Could you check a few things on this model? Use its own coordinates, in mm. A direction names the side the tool comes from. Give positions to 0.01 mm unless a question says otherwise; leave off trailing zeros. Order: outer loops, then holes, each group sorted by start corner. A loop starts at its lowest first (then second) coordinate and runs counter-clockwise, first axis right, second up. Notation, with made-up numbers: (-4.75, -21.5) -> (41.25, -21.5) arc R29 cw to (41.25, 8.5) -> close; hole circle Ø4 at (38, 60.5). An arc over 180 degrees is marked (long way). Write each question's results on one line, items separated by ' | '.
```python
from build123d import *

# Parameters (mm, degrees)
SKETCH_4_R          = 10
CUT_EXTRUDE_1_DEPTH = 40
CUT_EXTRUDE_5_DEPTH = 14
CUT_EXTRUDE_6_DEPTH = 14


with BuildPart() as part:
    # Sketch 1 → Revolve 1 (revolve)
    with BuildSketch(Plane.XY):
        Polygon((-131.316498316, -36.008306789), (-131.316498316, 163.991693211), (-116.316498316, 163.991693211), (-98.316498316, 133.991693211), (-64.316498316, 133.991693211), (-46.316498316, 163.991693211), (-31.316498316, 163.991693211), (-31.316498316, -36.008306789), align=None)
    revolve(axis=Axis((-31.316498316, -36.008306789, 0), (-1, 0, 0)))

    # Sketch 4 → Cut-Extrude 1 (cut)
    with BuildSketch(Plane.ZY.offset(131.316498316)):
        with Locations(Location((0, -36.008306789, 0), (0, 0, 270))):
            Circle(SKETCH_4_R)
    extrude(amount=-CUT_EXTRUDE_1_DEPTH, mode=Mode.SUBTRACT)

    # Sketch 9 → Cut-Extrude 5 (cut)
    with BuildSketch(Plane.XY):
        with BuildLine():
            Line((-101.316498316, -31.008306789), (-121.316498316, -31.008306789))
            ThreePointArc((-121.316498316, -31.008306789), (-117.780964411, -32.472772883), (-116.316498316, -36.008306789))
            ThreePointArc((-116.316498316, -36.008306789), (-117.780964411, -39.543840695), (-121.316498316, -41.008306789))
            Line((-121.316498316, -41.008306789), (-101.316498316, -41.008306789))
            ThreePointArc((-101.316498316, -41.008306789), (-106.316498316, -36.008306789), (-101.316498316, -31.008306789))
        make_face()
        with BuildLine():
            ThreePointArc((-96.316498316, -36.008306789), (-97.780964411, -32.472772883), (-101.316498316, -31.008306789))
            Line((-101.316498316, -31.008306789), (-101.316498316, -41.008306789))
            ThreePointArc((-101.316498316, -41.008306789), (-97.780964411, -39.543840695), (-96.316498316, -36.008306789))
        make_face()
        with BuildLine():
            Line((-101.316498316, -41.008306789), (-101.316498316, -31.008306789))
            ThreePointArc((-101.316498316, -31.008306789), (-106.316498316, -36.008306789), (-101.316498316, -41.008306789))
        make_face()
        with BuildLine():
            ThreePointArc((-116.316498316, -36.008306789), (-117.780964411, -32.472772883), (-121.316498316, -31.008306789))
            Line((-121.316498316, -31.008306789), (-121.316498316, -41.008306789))
            ThreePointArc((-121.316498316, -41.008306789), (-117.780964411, -39.543840695), (-116.316498316, -36.008306789))
        make_face()
        with BuildLine():
            Line((-121.316498316, -41.008306789), (-121.316498316, -31.008306789))
            ThreePointArc((-121.316498316, -31.008306789), (-126.316498316, -36.008306789), (-121.316498316, -41.008306789))
        make_face()
    extrude(amount=-CUT_EXTRUDE_5_DEPTH, mode=Mode.SUBTRACT)

    # Sketch 9_4 → Cut-Extrude 6 (cut)
    with BuildSketch(Plane.XY):
        with BuildLine():
            ThreePointArc((-121.316498316, -41.008306789), (-126.316498316, -36.008306789), (-121.316498316, -31.008306789))
            Line((-121.316498316, -31.008306789), (-131.316498316, -31.008306789))
            Line((-131.316498316, -31.008306789), (-131.316498316, -41.008306789))
            Line((-131.316498316, -41.008306789), (-121.316498316, -41.008306789))
        make_face()
    extrude(amount=-CUT_EXTRUDE_6_DEPTH, mode=Mode.SUBTRACT)


solid = part.part
```
Q1. Suppose I cut it at B-B on x = -125. Please give me the cut outline in (y, z), and give its area (3 significant figures).
Here are the results:
outline: circle Ø400 at (-36.01, 0); hole (-41.01, -14) -> (-31.01, -14) -> (-31.01, -8.66) arc R10 ccw (long way) to (-41.01, -8.66) -> close | area: 125,000 mm²
Q2. For faces 4 (the conical face through (-99.19, -172.07, 104.33)), 5 (the cylindrical face through (-123.711, 154.756, -60.075)), 6 (the cylindrical face through (-111.596, -34.707, 9.915)), which set-ups out of +Z, -Z, +X, -X, +Y, -Y let a thin tool reach every point of the face, with its end or its side?
Here are the results:
face 4: none | face 5: +X, -X | face 6: -X
Q3. Suppose I cut it at A-A on z = 0. Please give me the cut outline in (x, y).
Here are the results:
outline: (-131.32, -236.01) -> (-116.32, -236.01) -> (-98.32, -206.01) -> (-64.32, -206.01) -> (-46.32, -236.01) -> (-31.32, -236.01) -> (-31.32, 163.99) -> (-46.32, 163.99) -> (-64.32, 133.99) -> (-98.32, 133.99) -> (-116.32, 163.99) -> (-131.32, 163.99) -> (-131.32, -26.01) -> (-91.32, -26.01) -> (-91.32, -46.01) -> (-131.32, -46.01) -> close
Q4. I need wall thicknesses on line 1 along X through (y, z) = (-200.5, -113.5); line 2 along X through (y, z) = (-190, -119.5); line 3 along Y through (x, z) = (-114, 0). Which ranges of each line are inside material? Lowest first, please.
Here are the results:
line 1: x = -131.32 to -116.23, -46.41 to -31.32 | line 2: x = -131.32 to -113.27, -49.36 to -31.32 | line 3: y = -232.15 to -46.01, -26.01 to 160.13
Q5. Suppose I cut it at C-C on x = -76.5. Please give me the cut outline in (y, z).
Here are the results:
outline: circle Ø340 at (-36.01, 0)
Q6. Thinking about a two-plate mould opening in Y: for faces 1 (the flat face through (-114, -36, -14)), 2 (the cylindrical face through (-81.078, 126.141, -51.063)), 3 (the flat face through (-131.316, -33, 42)), which applies, +Y half, -Y half, draft (parallel to the pull), parting line (faces both ways), or undercut?
Here are the results:
face 1: undercut | face 2: parting line | face 3: draft
Q7. I'm going to push flat-ended pins straight in: pin 1 Ø5 at (x, y) = (-116, -75.5) entering from -Z; pin 2 Ø3 at (y, z) = (108.5, -139) entering from +X; pin 3 Ø1.6 at (x, z) = (-117.5, -12.5) entering from +Y; pin 4 Ø6 at (x, z) = (-107, -55.5) entering from -Y. Where does each tip first touch, or does it pass through?
Here are the results:
pin 1: stops at z = -196.55 | pin 2: stops at x = -31.32 | pin 3: stops at y = 163.65 | pin 4: stops at y = -217.25
